CAD build for the part. Positions are in the model's coordinates, mm. Face numbers are marked on the shaded views. A direction names the side the tool comes from. Give positions to 0.01 mm unless a question says otherwise; leave off trailing zeros. Order: outer loops, then holes, each group sorted by start corner. A loop starts at its lowest first (then second) coordinate and runs counter-clockwise, first axis right, second up.
Item 1: Two-plate mould, pull along Z, no slides. Class the marked faces 1, 2 and 3: released by +Z, released by -Z, zero draft, split by the parting line, or undercut.
Item 2: Band-saw the part on A-A on z = 0. Give the cut face in (x, y).
Item 3: Flat gauge pins, fed straight in: P1, Ø3, axis at y = -18, z = -4.5, coming from the -X side; P2, Ø6, axis at x = 0, z = 0, coming from the -Y side; P3, Ø2.5, axis at x = -6, y = -16, coming from the +Z side; P4, Ø4.5, axis at x = -7.5, y = -17, coming from the -Z side. Where does each tip first touch, or does it go through?
Item 4: Band-saw the part on D-D on y = -3.75. Give the cut face in (x, z).
Item 5: Band-saw the part on B-B on y = -17.5. Give the cut face in (x, z).
Item 6: Wall check: L1, parallel to Z at x = 0, y = -11; L2, parallel to Z at x = 5.5, y = -14; L3, parallel to Y at x = 9.75, z = -8.75. Give the ranges that are in metal, low to high.
Item 7: Band-saw the part on C-C on x = -0.5. Give the cut face in (y, z), plus the area to 3 significant figures.
Item 8: Which spindle directions (+Z, -Z, +X, -X, +Y, -Y) get a long thin tool onto all of the face, cutting with end or side? Do the marked faces 4, 5, 6 and 7. Say none if no direction does.
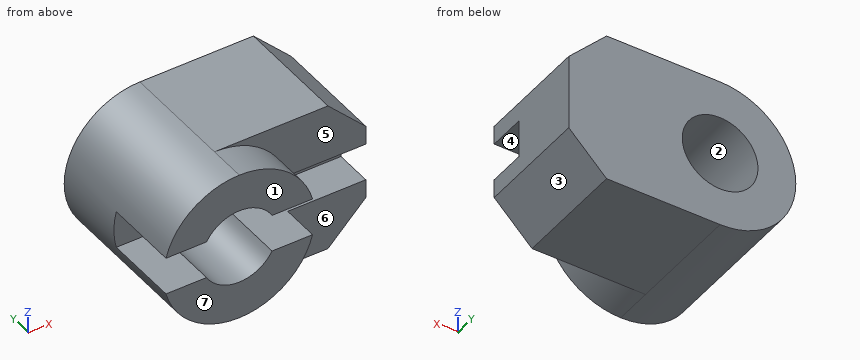
```python
from build123d import *

# Parameters (mm, degrees)
F1_DEPTH = 20
F2_DEPTH = 15
F3_R     = 5
F4_DEPTH = 20.001
F5_W     = 5
F5_H     = 5
F6_DEPTH = 30.001


with BuildPart() as f1:
    # F0 (on Front) → F1 (new body)
    with BuildSketch(Plane.XZ):
        with BuildLine():
            ThreePointArc((0, -10), (7.071068, -7.071068), (10, 0))
            ThreePointArc((10, 0), (7.071068, 7.071068), (0, 10))
            ThreePointArc((0, 10), (-10, 0), (0, -10))
        make_face()
    extrude(amount=F1_DEPTH)

    # F0 (on Front) → F2 (join)
    with BuildSketch(Plane.XZ):
        with BuildLine():
            ThreePointArc((0, 10), (7.071068, 7.071068), (10, 0))
            ThreePointArc((10, 0), (7.071068, -7.071068), (0, -10))
            Line((0, -10), (15, -10))
            Line((15, -10), (20, -5))
            Line((20, -5), (20, 5))
            Line((20, 5), (15, 10))
            Line((15, 10), (0, 10))
        make_face()
    extrude(amount=F2_DEPTH)

    # F3 (on face) → F4 (cut, through all)
    with BuildSketch(Plane.XZ.offset(20)):
        Circle(F3_R)
    extrude(amount=-F4_DEPTH, mode=Mode.SUBTRACT)

    # F5 (on face) → F6 (cut, through all)
    with BuildSketch(Plane.YZ.offset(20)):
        with Locations((-12.5, 0)):
            Rectangle(F5_W, F5_H)
        with Locations((-17.5, 0)):
            Rectangle(F5_W, F5_H)
    extrude(amount=-F6_DEPTH, mode=Mode.SUBTRACT)


solid = f1.part
```
The answers:
1. face 1: zero draft
1. face 2: undercut
1. face 3: released by -Z
2. outline: (-10, -10) - (-5, -10) - (-5, 0) - (-10, 0) - close; (5, -10) - (20, -10) - (20, 0) - (5, 0) - close
3. P1: stops at x = -9.54
3. P2: passes through
3. P3: stops at z = 8.8
3. P4: stops at z = -8.51
4. outline: (0, -10) - (15, -10) - (20, -5) - (20, 5) - (15, 10) - (0, 10) arc R10 ccw to start; hole circle Ø10 at (0, 0)
5. outline: (-9.68, -2.5) arc R10 ccw to (9.68, -2.5) - (4.33, -2.5) arc R5 cw to (-4.33, -2.5) - close; (-9.68, 2.5) - (-4.33, 2.5) arc R5 cw to (4.33, 2.5) - (9.68, 2.5) arc R10 ccw to start
6. L1: z = -10 to -5, 5 to 10
6. L2: z = -10 to -2.5, 2.5 to 10
6. L3: y = -15 to 0
7. outline: (-20, -9.99) - (0, -9.99) - (0, -4.97) - (-20, -4.97) - close; (-20, 4.97) - (0, 4.97) - (0, 9.99) - (-20, 9.99) - close
7. area: 201 mm2
8. face 4: +X, -X, -Y
8. face 5: +Z, +X, -Y
8. face 6: -Z, +X, -Y
8. face 7: +Z, -Z, +X, -X, -Y
